```python
from build123d import *


with BuildPart() as part:
    # Schizzo1 → Rivoluzione1 (revolve)
    with BuildSketch(Plane.XY):
        with BuildLine():
            Line((-2.911073127, 3.333333333), (-2.911073127, 2.666666667))
            Line((-2.911073127, 2.666666667), (-3.175073127, 2.666666667))
            Line((-3.175073127, 2.666666667), (-3.175073127, 2.150104382))
            Line((-3.175073127, 2.150104382), (-2.961146331, 2))
            Line((-2.961146331, 2), (-0.149968672, 2))
            Line((-0.149968672, 2), (-7.3127e-05, 2.150104382))
            Line((-7.3127e-05, 2.150104382), (-7.3127e-05, 2.666666667))
            Line((-7.3127e-05, 2.666666667), (-0.2, 2.666666667))
            Line((-0.2, 2.666666667), (-0.2, 3.333333333))
            Line((-0.2, 3.333333333), (-7.3127e-05, 3.333333333))
            Line((-7.3127e-05, 3.333333333), (-7.3127e-05, 4.5595))
            Line((-7.3127e-05, 4.5595), (-0.914073127, 4.5595))
            Line((-0.914073127, 4.5595), (-0.914073127, 4.02))
            ThreePointArc((-0.914073127, 4.02), (-0.899930992, 3.985857864), (-0.934073127, 4))
            Line((-0.934073127, 4), (-2.961, 4))
            Line((-2.961, 4), (-3.175073127, 3.850104382))
            Line((-3.175073127, 3.850104382), (-3.175073127, 3.333333333))
            Line((-3.175073127, 3.333333333), (-2.911073127, 3.333333333))
        make_face()
    revolve(axis=Axis((-4, 0, 0), (1, 0, 0)))


solid = part.part
```
Read the model definition and answer for the solid it produces. Units are mm, in the model's axes. A direction names the side the tool comes from. Give positions to 0.01 mm unless a question says otherwise; leave off trailing zeros. Loops run counter-clockwise (first coordinate to the right, second up) from the corner with the lowest first, then second, coordinate; pieces in that order, holes last.
Item 1: Find the intervals of material crossed by line 1 along Z through (x, y) = (-2.95, 0); line 2 along Z through (x, y) = (-3, 1); line 3 along Z through (x, y) = (-2.2, 0), in increasing order.
Item 2: Each of these flat-tipped pins is pushed along its axis until it touches: pin 1 Ø2.5 at (y, z) = (0, 0) entering from -X; pin 2 Ø1.5 at (x, z) = (-2, -0.5) entering from +Y. Where does it stop, or does it pass through?
Item 3: The part is cut by section A-A (x = -1.2). Write down the section's boundary in (y, z), and give its area (3 significant figures).
Item 4: For faces 1 (the flat face through (-0.2, 0, 3)), 2 (the flat face through (0, 2, -3)), 3 (the flat face through (-0.914, 3, -3)), determine the directions among +Z, -Z, +X, -X, +Y, -Y from which every point of the face is accessible in a straight line to the end or side of a thin tool.
Item 5: The mould has two halves that part along Z. Classify faces 4 (the cylindrical face through (-0.463, 2.451, 3.845)), 5 (the flat face through (-3.175, -3, 2)), 6 (the cylindrical face through (-2, 0, -2)): released by +Z, released by -Z, zero draft, split by the parting line, or undercut.
Taken from the geometry:
1. line 1: z = -4 to -3.33, -2.67 to -2, 2 to 2.67, 3.33 to 4
1. line 2: z = -3.84 to -3.18, -2.47 to -1.76, 1.76 to 2.47, 3.18 to 3.84
1. line 3: z = -4 to -2, 2 to 4
2. pin 1: passes through
2. pin 2: stops at y = 4
3. outline: circle Ø8 at (0, 0); hole circle Ø4 at (0, 0)
3. area: 37.7 mm2
4. face 1: +X
4. face 2: +Z, -Z, +X, +Y, -Y
4. face 3: -X
5. face 4: split by the parting line
5. face 5: zero draft
5. face 6: undercut
